The listing builds one solid part. Answer for the finished solid, in the listing's coordinates (mm). A direction names the side the tool comes from. Coordinates: 2 decimals unless noted, no trailing zeros. Write each loop counter-clockwise with the first axis right and the second up, starting at its lowest first coordinate (ties: lowest second). Pieces come first, ordered by that corner, then holes.
```python
from build123d import *

# Parameters (mm, degrees)
F0_W          = 65
F0_H          = 5
F1_ANGLE_BACK = 15
F1_ANGLE      = 30
F3_DEPTH      = 0.5
F5_D          = 8.4328


with BuildPart() as f1:
    # F0 (on Right) → F1 (revolve)
    with BuildSketch(Plane.YZ, mode=Mode.PRIVATE) as f1_sk:
        with Locations((32.5, 2.5)):
            Rectangle(F0_W, F0_H)
    revolve(f1_sk.sketch.rotate(Axis((0, -138, 18.1028265506), (0, 0, -1)), -F1_ANGLE_BACK), axis=Axis((0, -138, 18.1028265506), (0, 0, -1)), revolution_arc=F1_ANGLE)

    # F2 (on face) → F3 (cut)
    with BuildSketch(Plane(origin=(0, 0, 0), x_dir=(1, 0, 0), z_dir=(0, 0, -1))):
        Polygon((-17.7241188623, -71.9769457125), (-11.4765199745, 3e-10), (-11.9784, 3e-10), (-5.7345541206, 71.9337082881), (-6.2326811376, 71.9769457131), (-18.7203728964, -71.8904708623), align=None)
        Polygon((-11.9784, 3e-10), (-11.4765199745, 3e-10), (-5.2364271036, 71.890470863), (-5.7345541206, 71.9337082881), align=None)
        Polygon((-14.3904012595, -72.2317256548), (-9.2739048409, 3e-10), (-10.2764104633, 3e-10), (-15.3879018995, -72.1610682199), align=None)
        Polygon((-10.2764104633, 3e-10), (-9.2739048409, 3e-10), (-4.1868765839, 71.8157112602), (-5.184377224, 71.886368695), align=None)
        Polygon((-11.05306095, -72.4335808844), (-7.0761095593, 3e-10), (-8.0776156937, 3e-10), (-12.0515570806, -72.3787586524), align=None)
        Polygon((-8.0776156937, 3e-10), (-7.0761095593, 3e-10), (-3.1362720404, 71.7576131981), (-4.1347681711, 71.8124354301), align=None)
        Polygon((-7.7129380916, -72.5824605854), (-4.8820145346, 3e-10), (-5.8827748571, 3e-10), (-8.7121783467, -72.5434873575), align=None)
        Polygon((-5.8827748571, 3e-10), (-4.8820145346, 3e-10), (-2.0848779572, 71.7161913026), (-3.0841182124, 71.7551645305), align=None)
        Polygon((-4.3708735422, -72.678327278), (-2.6905077568, 3e-10), (-3.6907750019, 3e-10), (-5.3706063685, -72.6552128656), align=None)
        Polygon((-3.6907750019, 3e-10), (-2.6905077568, 3e-10), (-1.0329590172, 71.6914560015), (-2.0326918435, 71.714570414), align=None)
        Polygon((-1.0277086488, -72.7211568285), (-0.5004825388, 3e-10), (-1.5005088195, 3e-10), (-2.0276823688, -72.7139070503), align=None)
        Polygon((-1.5005088195, 3e-10), (-0.5004825388, 3e-10), (0.0192199648, 71.6834135218), (-0.9807537552, 71.6906633), align=None)
        Polygon((5.3267903546, 71.8976905392), (11.6665424492, 3e-10), (18.0111294073, -71.9525216273), (19.0072643041, -71.8646850327), (6.3229252514, 71.9855271339), align=None)
        Polygon((4.2773430078, 71.8214963276), (9.4634593874, 3e-10), (10.4660630255, 3e-10), (5.274746131, 71.8935172258), align=None)
        Polygon((10.4660630255, 3e-10), (9.4634593874, 3e-10), (14.6777631894, -72.2118583428), (15.6751663126, -72.1398374447), align=None)
        Polygon((3.2268188627, 71.7619622003), (7.2652930626, 3e-10), (8.2668753034, 3e-10), (4.2252391215, 71.8181492712), align=None)
        Polygon((8.2668753034, 3e-10), (7.2652930626, 3e-10), (11.3407019231, -72.4182753472), (12.3391221818, -72.3620882763), align=None)
        Polygon((2.1754823833, 71.7191031448), (5.0709231192, 3e-10), (6.071737735, 3e-10), (3.1746684306, 71.7594422436), align=None)
        Polygon((6.071737735, 3e-10), (5.0709231192, 3e-10), (8.0007856957, -72.571720676), (8.999971743, -72.5313815772), align=None)
        Polygon((1.1235982379, 71.6929299507), (2.8792369834, 3e-10), (3.8795367771, 3e-10), (2.123298534, 71.7174109221), align=None)
        Polygon((3.8795367771, 3e-10), (2.8792369834, 3e-10), (4.6588553133, -72.6721557002), (5.6585556094, -72.6476747287), align=None)
        Polygon((0.0714312325, 71.6834492068), (0.6891275978, 3e-10), (1.6891647234, 3e-10), (1.0713941082, 71.6920658881), align=None)
        Polygon((1.6891647234, 3e-10), (0.6891275978, 3e-10), (1.315752089, -72.7195551358), (2.3157149647, -72.7109384546), align=None)
    extrude(amount=-F3_DEPTH, mode=Mode.SUBTRACT)

    # F5 (through all)
    with Locations(Plane(origin=(0, 0, 0), x_dir=(1, 0, 0), z_dir=(0, 0, -1))):
        with Locations((-30.363664634, -4.2965139067), (30.363664634, -4.2965139067), (43.3174317129, -52.6406307947), (-43.3174317129, -52.6406307947)):
            Hole(F5_D / 2)


solid = f1.part
```
(1) Section A-A, the plane x = -45.5 is taken. Write down the section's boundary in (y, z).
(2) Each of these flat-tipped pins is pushed along its axis until it touches: pin 1 (7.5 mm diameter, centred on x = -30.36, y = 4.3, fed in from -Z); pin 2 (2 mm diameter, centred on y = 35.5, z = 2.5, fed in from -X); pin 3 (1.5 mm diameter, centred on y = 6.5, z = 1, fed in from -X); pin 4 (1 mm diameter, centred on y = 16, z = 2.5, fed in from -X). Where does it stop, or does it pass through?
(3) For a pull along Y with two mould halves and no side action, classify faces 1 (the flat face through (-15.203, 31.364, 0.246)), 2 (the cylindrical face through (26.47, 5.91, 2.53)), 3 (the flat face through (-44.01, 26.25, 2.54)), 4 (the flat face through (6, 35, 0)) as pulls with the +Y half, pulls with the -Y half, needs draft (parallel to the pull), parting line crosses it, or undercut.
(4) Section D-D, the plane x = 33.5 is taken. Write down the section's boundary in (y, z), plus the area to 3 significant figures.
(5) Section B-B, the plane z = 3.6 is taken. Write down the section's boundary in (x, y), plus the area to 3 significant figures.
(6) Section C-C, the plane y = 54.5 is taken. State how many separate pieces and enclosed holes the cut face has, plus the area to 3 significant figures.
(7) Find the intervals of material crossed by probe 1 along X at (y, z) = (0.5, 4.45); probe 2 along Y at (x, z) = (-1.5, 3.95); probe 3 along Y at (x, z) = (5.5, 3.9), in increasing order.
(8) Which of the six approach directions +Z, -Z, +X, -X, +Y, -Y give full straight-line access (tool end or side, diameter ignored) to faces 5 (the flat face through (-11, 35, 0)), 6 (the flat face through (-7, 35, 0.5))?
Solution:
1. outline: (31.81, 0) - (49.03, 0) - (49.03, 5) - (31.81, 5) - close; (56.25, 0) - (59.84, 0) - (59.84, 5) - (56.25, 5) - close
2. pin 1: passes through
2. pin 2: stops at x = -46.76
2. pin 3: stops at x = -38.92
2. pin 4: stops at x = -41.4
3. face 1: undercut
3. face 2: undercut
3. face 3: pulls with the -Y half
3. face 4: needs draft
4. outline: (-4.13, 0) - (1.48, 0) - (1.48, 5) - (-4.13, 5) - close; (7.11, 0) - (62.22, 0) - (62.22, 5) - (7.11, 5) - close
4. area: 304 mm2
5. outline: (-52.54, 58.08) - (-35.72, -4.7) arc R138 cw to (35.72, -4.7) - (52.54, 58.08) arc R203 ccw to start; hole circle Ø8.43 at (-43.32, 52.64); hole circle Ø8.43 at (-30.36, 4.3); hole circle Ø8.43 at (30.36, 4.3); hole circle Ø8.43 at (43.32, 52.64)
5. area: 5,580 mm2
6. separate pieces: 3
6. enclosed holes: 0
6. area: 434 mm2
7. probe 1: x = -37.11 to -32.2, -28.53 to 28.53, 32.2 to 37.11
7. probe 2: y = -0.01 to 64.99
7. probe 3: y = -0.11 to 64.93
8. face 5: -Z, +X, -X, +Y, -Y
8. face 6: -Z
